Part model, mm, in its own coordinate system. A direction names the side the tool comes from. Coordinates: 2 decimals unless noted, no trailing zeros. Write each loop counter-clockwise with the first axis right and the second up, starting at its lowest first coordinate (ties: lowest second). Pieces come first, ordered by that corner, then holes. Notation, with made-up numbers: (68.25, 83.25) -> (98.25, 83.25) arc R12 ccw to (98.25, 106.25) -> close; hole circle Ø10 at (13.25, 38). An arc over 180 degrees is marked (long way). Write item = value, one per line.
from build123d import *

# Parameters (mm, degrees)
ESQUISSE1_R        = 1.75
BOSS_EXTRU_1_DEPTH = 5
ESQUISSE2_R        = 3.5
BOSS_EXTRU_2_DEPTH = 2
CONG_1_R           = 1


with BuildPart() as part:
    # Esquisse1 → Boss.-Extru.1 (new body)
    with BuildSketch(Plane(origin=(0, 0, 0), x_dir=(1, 0, 0), z_dir=(0, 1, 0))):
        with Locations(Location((0, 0, 0), (0, 0, 270))):
            Circle(ESQUISSE1_R)
    extrude(amount=BOSS_EXTRU_1_DEPTH)

    # Esquisse2 → Boss.-Extru.2 (add)
    with BuildSketch(Plane(origin=(0, 5, 0), x_dir=(1, 0, 0), z_dir=(0, 1, 0))):
        with Locations(Location((0, 0, 0), (0, 0, 270))):
            Circle(ESQUISSE2_R)
    extrude(amount=BOSS_EXTRU_2_DEPTH)

    # Cong_1
    cong_1_edges = [part.edges().sort_by_distance(p)[0] for p in [
        (0, 7, -3.5),
    ]]
    fillet(cong_1_edges, radius=CONG_1_R)


solid = part.part
Q1. Probe line 1 (Y direction, x = -0.25, z = -2.5); line 2 (X direction, y = 2, z = 0); line 3 (Z direction, x = -2.5, y = 6). List the from-to ranges inside material, lowest first. Write a range as from..to.
Model answer:
line_1 = 5..7
line_2 = -1.75..1.75
line_3 = -2.45..2.45
Q2. Saw through at B-B on x = 0. Give the cut face in (y, z).
Model answer:
outline = (0, -1.75) -> (5, -1.75) -> (5, -3.5) -> (6, -3.5) arc R1 ccw to (7, -2.5) -> (7, 2.5) arc R1 ccw to (6, 3.5) -> (5, 3.5) -> (5, 1.75) -> (0, 1.75) -> close
Q3. Saw through at A-A on z = 0. Give the cut face in (x, y), and give its area (3 significant figures).
Model answer:
outline = (-3.5, 5) -> (-1.75, 5) -> (-1.75, 0) -> (1.75, 0) -> (1.75, 5) -> (3.5, 5) -> (3.5, 6) arc R1 ccw to (2.5, 7) -> (-2.5, 7) arc R1 ccw to (-3.5, 6) -> close
area = 31.1 mm²
Q4. Saw through at D-D on y = 0.5. Give the cut face in (x, z).
Model answer:
outline = circle Ø3.5 at (0, 0)
Q5. Which spindle directions (+Z, -Z, +X, -X, +Y, -Y) get a long thin tool onto all of the face, cutting with end or side? Do faces 1 (the face through (2, 5, 1)), 2 (the face through (-3.417, 5.493, -0.759)). Say none if no direction does.
Model answer:
face_1 = -Y
face_2 = +Y, -Y
Q6. Saw through at C-C on y = 5.5. Give the cut face in (x, z).
Model answer:
outline = circle Ø7 at (0, 0)
Q7. Pin check, flat tip, straight feed: pin 1 (3.5 mm diameter, centred on x = 1.5, z = 1, fed in from -Y). Stop position of the tip, or through.
Model answer:
pin_1 = 0
